Here's how the part is built. I have some questions about the finished solid (model axes, mm). Give positions to 0.01 mm unless a question says otherwise; leave off trailing zeros. Loops run counter-clockwise (first coordinate to the right, second up) from the corner with the lowest first, then second, coordinate; pieces in that order, holes last. Notation, with made-up numbers: (66, 56.25) - (109, 56.25) arc R14 cw to (109, 83.25) - close; hole circle Ø5 at (-34.75, 82). An arc over 180 degrees is marked (long way). Return JSON: item names as keys, results as strings. Group by question number.
(1) I need wall thicknesses on probe 1 along X at (y, z) = (-18.5, 0.65); probe 2 along Y at (x, z) = (91, 2.55); probe 3 along Y at (x, z) = (-33.5, 1.6). Which ranges of each line are inside material? Lowest first, please. Write a range as [from, to].
(2) For P1, Ø13, axis at x = 184.19, y = 10, coming from the -Z side, with a flat end and sliding along its axis, tell me the tip position at first contact or that it passes through.
(3) If we mould it in two halves opening along Y, with no side actions, what happens to faces 1 (the cylindrical face through (66.865, 12.418, 2.465)), 2 (the flat face through (106, 0, 0)), 3 (the cylindrical face through (191.623, 6.917, 2.465))? For each: released by +Y, released by -Y, zero draft, split by the parting line, or undercut.
(4) If we section it at C-C (x = 61): Please give me the cut outline in (y, z).
(5) If we section it at A-A (x = 12): Please give me the cut outline in (y, z).
(6) If we section it at B-B (z = 4.2): State how many separate pieces and enclosed holes the cut face has, then the cut area to 3 significant figures.
```python
from build123d import *

# Parameters (mm, degrees)
SKETCH1_W           = 390
SKETCH1_H           = 45
SKETCH1_R           = 8.05
SKETCH1_R_2         = 1.5
SKETCH1_W_2         = 5
SKETCH1_H_2         = 10
BOSS_EXTRUDE1_DEPTH = 5


with BuildPart() as part:
    # Sketch1 → Boss-Extrude1 (new body)
    with BuildSketch(Plane.XY):
        with Locations((109.186746988, 0)):
            Rectangle(SKETCH1_W, SKETCH1_H)
        with Locations((-65.813253012, 10)):
            Circle(SKETCH1_R, mode=Mode.SUBTRACT)
        with Locations((-40.813253012, 10)):
            Circle(SKETCH1_R, mode=Mode.SUBTRACT)
        with Locations((-15.813253012, 10)):
            Circle(SKETCH1_R, mode=Mode.SUBTRACT)
        with Locations((9.186746988, 10)):
            Circle(SKETCH1_R, mode=Mode.SUBTRACT)
        with Locations((34.186746988, 10)):
            Circle(SKETCH1_R, mode=Mode.SUBTRACT)
        with Locations((59.186746988, 10)):
            Circle(SKETCH1_R, mode=Mode.SUBTRACT)
        with Locations((84.186746988, 10)):
            Circle(SKETCH1_R, mode=Mode.SUBTRACT)
        with Locations((109.186746988, 10)):
            Circle(SKETCH1_R, mode=Mode.SUBTRACT)
        with Locations((134.186746988, 10)):
            Circle(SKETCH1_R, mode=Mode.SUBTRACT)
        with Locations((159.186746988, 10)):
            Circle(SKETCH1_R, mode=Mode.SUBTRACT)
        with Locations((184.186746988, 10)):
            Circle(SKETCH1_R, mode=Mode.SUBTRACT)
        with Locations((209.186746988, 10)):
            Circle(SKETCH1_R, mode=Mode.SUBTRACT)
        with Locations((234.186746988, 10)):
            Circle(SKETCH1_R, mode=Mode.SUBTRACT)
        with Locations((259.186746988, 10)):
            Circle(SKETCH1_R, mode=Mode.SUBTRACT)
        with Locations((284.186746988, 10)):
            Circle(SKETCH1_R, mode=Mode.SUBTRACT)
        with Locations(Location((284.186746988, -10, 0), (0, 0, 180))):
            Circle(SKETCH1_R, mode=Mode.SUBTRACT)
        with Locations(Location((259.186746988, -10, 0), (0, 0, 180))):
            Circle(SKETCH1_R, mode=Mode.SUBTRACT)
        with Locations(Location((234.186746988, -10, 0), (0, 0, 180))):
            Circle(SKETCH1_R, mode=Mode.SUBTRACT)
        with Locations(Location((209.186746988, -10, 0), (0, 0, 180))):
            Circle(SKETCH1_R, mode=Mode.SUBTRACT)
        with Locations(Location((184.186746988, -10, 0), (0, 0, 180))):
            Circle(SKETCH1_R, mode=Mode.SUBTRACT)
        with Locations(Location((159.186746988, -10, 0), (0, 0, 180))):
            Circle(SKETCH1_R, mode=Mode.SUBTRACT)
        with Locations(Location((134.186746988, -10, 0), (0, 0, 180))):
            Circle(SKETCH1_R, mode=Mode.SUBTRACT)
        with Locations(Location((109.186746988, -10, 0), (0, 0, 180))):
            Circle(SKETCH1_R, mode=Mode.SUBTRACT)
        with Locations(Location((84.186746988, -10, 0), (0, 0, 180))):
            Circle(SKETCH1_R, mode=Mode.SUBTRACT)
        with Locations(Location((59.186746988, -10, 0), (0, 0, 180))):
            Circle(SKETCH1_R, mode=Mode.SUBTRACT)
        with Locations(Location((34.186746988, -10, 0), (0, 0, 180))):
            Circle(SKETCH1_R, mode=Mode.SUBTRACT)
        with Locations(Location((9.186746988, -10, 0), (0, 0, 180))):
            Circle(SKETCH1_R, mode=Mode.SUBTRACT)
        with Locations(Location((-15.813253012, -10, 0), (0, 0, 180))):
            Circle(SKETCH1_R, mode=Mode.SUBTRACT)
        with Locations(Location((-40.813253012, -10, 0), (0, 0, 180))):
            Circle(SKETCH1_R, mode=Mode.SUBTRACT)
        with Locations(Location((-65.813253012, -10, 0), (0, 0, 180))):
            Circle(SKETCH1_R, mode=Mode.SUBTRACT)
        with Locations((-78.313253012, 0)):
            Circle(SKETCH1_R_2, mode=Mode.SUBTRACT)
        with Locations(Location((296.686746988, 0, 0), (0, 0, 180))):
            Circle(SKETCH1_R_2, mode=Mode.SUBTRACT)
        with Locations((-78.313253012, -15)):
            Rectangle(SKETCH1_W_2, SKETCH1_H_2, mode=Mode.SUBTRACT)
        with Locations((-78.313253012, 15)):
            Rectangle(SKETCH1_W_2, SKETCH1_H_2, mode=Mode.SUBTRACT)
        with Locations((296.686746988, -15)):
            Rectangle(SKETCH1_W_2, SKETCH1_H_2, mode=Mode.SUBTRACT)
        with Locations((296.686746988, 15)):
            Rectangle(SKETCH1_W_2, SKETCH1_H_2, mode=Mode.SUBTRACT)
    extrude(amount=BOSS_EXTRUDE1_DEPTH)


solid = part.part
```
Values:
{
 "1": {"probe 1": "[-85.81, -80.81], [-75.81, 294.19], [299.19, 304.19]", "probe 2": "[-22.5, -14.29], [-5.71, 5.71], [14.29, 22.5]", "probe 3": "[-22.5, -13.36], [-6.64, 6.64], [13.36, 22.5]"},
 "2": {"P1": "through"},
 "3": {"face 1": "undercut", "face 2": "zero draft", "face 3": "undercut"},
 "4": {"outline": "(-22.5, 0) - (-17.84, 0) - (-17.84, 5) - (-22.5, 5) - close; (-2.16, 0) - (2.16, 0) - (2.16, 5) - (-2.16, 5) - close; (17.84, 0) - (22.5, 0) - (22.5, 5) - (17.84, 5) - close"},
 "5": {"outline": "(-22.5, 0) - (-17.54, 0) - (-17.54, 5) - (-22.5, 5) - close; (-2.46, 0) - (2.46, 0) - (2.46, 5) - (-2.46, 5) - close; (17.54, 0) - (22.5, 0) - (22.5, 5) - (17.54, 5) - close"},
 "6": {"separate pieces": "1", "enclosed holes": "36", "area": "11,200 mm2"}
}
